Work out the finished part from the listing and answer in its coordinate system (mm). Face numbers are marked on the shaded views. A direction names the side the tool comes from. Give positions to 0.01 mm unless a question says otherwise; leave off trailing zeros. Write each loop counter-clockwise with the first axis right and the second up, starting at its lowest first coordinate (ties: lowest second). Pieces come first, ordered by that corner, then holes. Notation, with made-up numbers: (31.5, 76) -> (49.5, 76) arc R28 ccw to (49.5, 100) -> close; hole circle Ø7 at (6.25, 72). An arc over 180 degrees is marked (long way). Use a Markdown table: item, result. Add a question column.
Q1. Section B-B, the plane y = 10.25 is taken. Give the vertices of the cut face in (x, z).
Q2. Section C-C, the plane x = -0.75 is taken. Give the vertices of the cut face in (y, z).
Q3. Each of these flat-tipped pins is pushed along its axis until it touches: pin 1 Ø2.5 at (y, z) = (5.5, 22.5) entering from -X; pin 2 Ø1.5 at (x, z) = (7, 9) entering from -Y; pin 3 Ø1.5 at (y, z) = (5, 36.5) entering from -X; pin 4 Ø0.9 at (x, z) = (11, 40.5) entering from +Y. Where does it stop, or does it pass through?
Q4. Consider line 1 (Y direction, x = 4.25, z = 9.75); line 2 (Y direction, x = 6.5, z = 5.5); line 3 (Z direction, x = 12.85, y = 1.8). Determine where each line is inside the solid, lowest interval first.
Q5. For the marked faces 1, 2 and 3, determine the directions among +Z, -Z, +X, -X, +Y, -Y from which every point of the face is accessible in a straight line to the end or side of a thin tool.
Q6. Section D-D, the plane z = 9.75 is taken. Give the vertices of the cut face in (x, y).
Q7. Section A-A, the plane z = 40 is taken. Give the vertices of the cut face in (x, y).
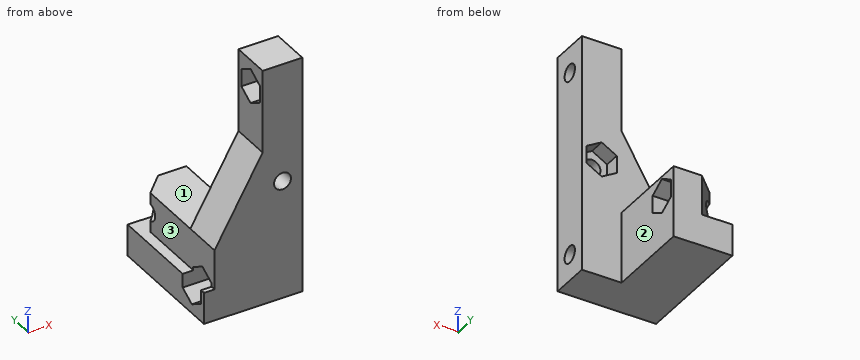
from build123d import *

# Parameters (mm, degrees)
SALIENTE_EXTRUIR1_DEPTH = 6
SALIENTE_EXTRUIR2_DEPTH = 7.5
SALIENTE_EXTRUIR3_DEPTH = 7.5
CROQUIS4_W              = 7.5
CROQUIS4_H              = 7.5
SALIENTE_EXTRUIR4_DEPTH = 31.5
CORTAR_EXTRUIR1_REACH   = 20.6
CROQUIS5_R              = 1.6
CORTAR_EXTRUIR2_DEPTH   = 14.1
CORTAR_EXTRUIR3_DEPTH   = 3
CORTAR_EXTRUIR4_REACH   = 25.65
CROQUIS8_R              = 1.6
CORTAR_EXTRUIR5_DEPTH   = 3
CORTAR_EXTRUIR6_REACH   = 13.1
CROQUIS10_R             = 1.6
CORTAR_EXTRUIR7_DEPTH   = 3


with BuildPart() as part:
    # Croquis1 → Saliente-Extruir1 (new body)
    with BuildSketch(Plane.XY):
        Polygon((0, 0), (16.6, 0), (16.6, 7.5), (9.1, 7.5), (9.1, 23.65), (3.75, 23.65), (-2, 23.65), (-2, 0), align=None)
    extrude(amount=SALIENTE_EXTRUIR1_DEPTH)

    # Croquis2 → Saliente-Extruir2 (add)
    with BuildSketch(Plane.XY.offset(6)):
        Polygon((0, 0), (0, 19.9), (3.75, 23.65), (9.1, 23.65), (9.1, 7.5), (16.6, 7.5), (16.6, 0), align=None)
    extrude(amount=SALIENTE_EXTRUIR2_DEPTH)

    # Croquis3 → Saliente-Extruir3 (add)
    with BuildSketch(Plane.XZ):
        Polygon((0, 13.5), (9.1, 29.261662349), (9.1, 13.5), align=None)
    extrude(amount=-SALIENTE_EXTRUIR3_DEPTH)

    # Croquis4 → Saliente-Extruir4 (add)
    with BuildSketch(Plane.XY.offset(13.5)):
        with Locations((12.85, 3.75)):
            Rectangle(CROQUIS4_W, CROQUIS4_H)
    extrude(amount=SALIENTE_EXTRUIR4_DEPTH)

    # Croquis5 → Cortar-Extruir1 (cut, up to next)
    with BuildSketch(Plane(origin=(16.6, 0, 0), x_dir=(0, 0, -1), z_dir=(1, 0, 0)), mode=Mode.PRIVATE) as cortar_extruir1_sk1:
        with Locations((-5, 3.75)):
            Circle(CROQUIS5_R)
    cortar_extruir1_tool1 = extrude(cortar_extruir1_sk1.sketch, amount=-CORTAR_EXTRUIR1_REACH, mode=Mode.PRIVATE) & part.part
    add(cortar_extruir1_tool1.solids().sort_by_distance((16.6, 3.75, 5))[0], mode=Mode.SUBTRACT)
    # Croquis5 → Cortar-Extruir1 (cut, up to next)
    with BuildSketch(Plane(origin=(16.6, 0, 0), x_dir=(0, 0, -1), z_dir=(1, 0, 0)), mode=Mode.PRIVATE) as cortar_extruir1_sk2:
        with Locations((-40, 3.75)):
            Circle(CROQUIS5_R)
    cortar_extruir1_tool2 = extrude(cortar_extruir1_sk2.sketch, amount=-CORTAR_EXTRUIR1_REACH, mode=Mode.PRIVATE) & part.part
    add(cortar_extruir1_tool2.solids().sort_by_distance((16.6, 3.75, 40))[0], mode=Mode.SUBTRACT)

    # Croquis6 → Cortar-Extruir2 (cut)
    with BuildSketch(Plane.ZY.offset(2)):
        Polygon((3.354551733, 0.9), (6.645448267, 0.9), (8.290896534, 3.75), (6.645448267, 6.6), (3.354551733, 6.6), (1.709103466, 3.75), align=None)
    extrude(amount=-CORTAR_EXTRUIR2_DEPTH, mode=Mode.SUBTRACT)

    # Croquis7 → Cortar-Extruir3 (cut)
    with BuildSketch(Plane.ZY.offset(-9.1)):
        Polygon((38.354551733, 0.9), (41.645448267, 0.9), (43.290896534, 3.75), (41.645448267, 6.6), (38.354551733, 6.6), (36.709103466, 3.75), align=None)
    extrude(amount=-CORTAR_EXTRUIR3_DEPTH, mode=Mode.SUBTRACT)

    # Croquis8 → Cortar-Extruir4 (cut, up to next)
    with BuildSketch(Plane.XZ, mode=Mode.PRIVATE) as cortar_extruir4_sk1:
        with Locations((12.85, 22.5)):
            Circle(CROQUIS8_R)
    cortar_extruir4_tool1 = extrude(cortar_extruir4_sk1.sketch, amount=-CORTAR_EXTRUIR4_REACH, mode=Mode.PRIVATE) & part.part
    add(cortar_extruir4_tool1.solids().sort_by_distance((12.85, 0, 22.5))[0], mode=Mode.SUBTRACT)

    # Croquis9 → Cortar-Extruir5 (cut)
    with BuildSketch(Plane(origin=(0, 7.5, 0), x_dir=(1, 0, 0), z_dir=(0, 1, 0))):
        Polygon((15.7, -20.854551733), (12.85, -19.209103466), (10, -20.854551733), (10, -24.145448267), (12.85, -25.790896534), (15.7, -24.145448267), align=None)
    extrude(amount=-CORTAR_EXTRUIR5_DEPTH, mode=Mode.SUBTRACT)

    # Croquis10 → Cortar-Extruir6 (cut, up to next)
    with BuildSketch(Plane(origin=(9.1, 0, 0), x_dir=(0, 0, -1), z_dir=(1, 0, 0)), mode=Mode.PRIVATE) as cortar_extruir6_sk1:
        with Locations((-9.75, 20)):
            Circle(CROQUIS10_R)
    cortar_extruir6_tool1 = extrude(cortar_extruir6_sk1.sketch, amount=-CORTAR_EXTRUIR6_REACH, mode=Mode.PRIVATE) & part.part
    add(cortar_extruir6_tool1.solids().sort_by_distance((9.1, 20, 9.75))[0], mode=Mode.SUBTRACT)

    # Croquis11 → Cortar-Extruir7 (cut)
    with BuildSketch(Plane(origin=(9.1, 0, 0), x_dir=(0, 0, -1), z_dir=(1, 0, 0))):
        Polygon((-8.104551733, 22.85), (-11.395448267, 22.85), (-13.040896534, 20), (-11.395448267, 17.15), (-8.104551733, 17.15), (-6.459103466, 20), align=None)
    extrude(amount=-CORTAR_EXTRUIR7_DEPTH, mode=Mode.SUBTRACT)


solid = part.part
Result set:
| question | item | result |
|---|---|---|
| 1 | outline | (-2, 0) -> (9.1, 0) -> (9.1, 13.5) -> (0, 13.5) -> (0, 6) -> (-2, 6) -> close |
| 2 | outline | (0, 0) -> (23.65, 0) -> (23.65, 6) -> (6.6, 6) -> (6.6, 3.35) -> (3.75, 1.71) -> (0.9, 3.35) -> (0.9, 6) -> (0, 6) -> close |
| 3 | pin 1 | stops at x = 4.47 |
| 3 | pin 2 | stops at y = 0 |
| 3 | pin 3 | stops at x = 9.1 |
| 3 | pin 4 | stops at y = 7.5 |
| 4 | line 1 | y = 0 to 18.4, 21.6 to 23.65 |
| 4 | line 2 | y = 0 to 0.9, 6.6 to 23.65 |
| 4 | line 3 | z = 0 to 20.9, 24.1 to 45 |
| 5 | face 1 | +Z, +X, -X, +Y |
| 5 | face 2 | +Z, -Z, +X, +Y |
| 5 | face 3 | +Z, -X, +Y, -Y |
| 6 | outline | (0, 0) -> (16.6, 0) -> (16.6, 7.5) -> (9.1, 7.5) -> (9.1, 17.15) -> (6.1, 17.15) -> (6.1, 18.4) -> (0, 18.4) -> close; (1.7, 21.6) -> (6.1, 21.6) -> (6.1, 22.85) -> (9.1, 22.85) -> (9.1, 23.65) -> (3.75, 23.65) -> close |
| 7 | outline | (9.1, 0) -> (16.6, 0) -> (16.6, 2.15) -> (12.1, 2.15) -> (12.1, 0.9) -> (9.1, 0.9) -> close; (9.1, 6.6) -> (12.1, 6.6) -> (12.1, 5.35) -> (16.6, 5.35) -> (16.6, 7.5) -> (9.1, 7.5) -> close |
